Read the model definition and answer for the solid it produces. Units are mm, in the model's axes. Face numbers are marked on the shaded views. A direction names the side the tool comes from. Coordinates: 2 decimals unless noted, no trailing zeros. Write each loop counter-clockwise with the first axis right and the second up, starting at its lowest first coordinate (ties: lowest second). Pieces come first, ordered by that corner, then holes. Notation, with made-up numbers: (39.5, -1) -> (58.5, -1) arc R19 cw to (58.5, 36) -> close; hole circle Ø7 at (73.25, 55). An arc over 180 degrees is marked (long way). Answer as a JSON object with one key per item and string values. Group by question number.
(1) Find section B-B (z = 12.5). Give the vertices of the cut face in (x, y).
(2) Flat-ended cylindrical pins translate along their axes: P1, Ø12, axis at x = 38, z = 14.5, coming from the +Y side; P2, Ø6, axis at x = -20.5, y = 8.5, coming from the +Z side; P3, Ø4.5, axis at x = 6, z = -6, coming from the +Y side. Find the tip coordinate at first contact, or state that the pin passes through.
(3) Which of the six approach directions +Z, -Z, +X, -X, +Y, -Y give full straight-line access (tool end or side, diameter ignored) to the marked faces 5, 6, 7, 8 and 9?
(4) For a pull along X with two mould halves and no side action, classify the marked faces 1, 2, 3 and 4 as +X half, -X half, draft (parallel to the pull), parting line (faces both ways), or undercut.
(5) Straight lines are drawn through the part: L1, parallel to X at y = 15, z = -7; L2, parallel to X at y = 17, z = -8.5; L3, parallel to X at y = 1.5, z = -0.5. For each, find the intervals that lie inside material, in ascending order.
(6) Find section C-C (y = -24). Give the vertices of the cut face in (x, z), then the cut area to 3 significant figures.
(7) Find section D-D (y = 15). Give the vertices of the cut face in (x, z).
(8) Find section A-A (x = -37.5). Give the vertices of the cut face in (y, z), then the cut area to 3 significant figures.
from build123d import *

# Parameters (mm, degrees)
BOSS_EXTRUDE1_DEPTH = 15
SKETCH2_W           = 25
SKETCH2_H           = 10
BOSS_EXTRUDE2_DEPTH = 25
SKETCH3_R           = 2
CUT_EXTRUDE1_DEPTH  = 10


with BuildPart() as part:
    # Sketch1 → Boss-Extrude1 (new body)
    with BuildSketch(Plane.XY):
        with BuildLine():
            Line((-15, 0), (0, 0))
            Line((0, 0), (15, 0))
            Line((15, 0), (15, 30))
            Line((15, 30), (26.540029545, 30))
            Line((26.540029545, 30), (26.540029545, 18.872983346))
            ThreePointArc((26.540029545, 18.872983346), (27.540029545, 11), (28.540029545, 18.872983346))
            Line((28.540029545, 18.872983346), (28.540029545, 30))
            Line((28.540029545, 30), (40, 30))
            Line((40, 30), (40, 0))
            Line((40, 0), (50, -20))
            Line((50, -20), (50, -30))
            Line((50, -30), (0, -30))
            Line((0, -30), (-50, -30))
            Line((-50, -30), (-50, -20))
            Line((-50, -20), (-40, 0))
            Line((-40, 0), (-40, 30))
            Line((-40, 30), (-28.459970455, 30))
            Line((-28.459970455, 30), (-28.459970455, 18.872983346))
            ThreePointArc((-28.459970455, 18.872983346), (-27.459970455, 11), (-26.459970455, 18.872983346))
            Line((-26.459970455, 18.872983346), (-26.459970455, 30))
            Line((-26.459970455, 30), (-15, 30))
            Line((-15, 30), (-15, 0))
        make_face()
    extrude(amount=-BOSS_EXTRUDE1_DEPTH)

    # Sketch2 → Boss-Extrude2 (add)
    with BuildSketch(Plane.XY):
        with Locations((-37.5, -25)):
            Rectangle(SKETCH2_W, SKETCH2_H)
        with Locations((37.5, -25)):
            Rectangle(SKETCH2_W, SKETCH2_H)
    extrude(amount=BOSS_EXTRUDE2_DEPTH)

    # Sketch3 → Cut-Extrude1 (cut)
    with BuildSketch(Plane(origin=(0, -20, 0), x_dir=(1, 0, 0), z_dir=(0, 1, 0))):
        with Locations(Location((-37.5, -12.5, 0), (0, 0, 270))):
            Circle(SKETCH3_R)
        with Locations(Location((37.5, -12.5, 0), (0, 0, 270))):
            Circle(SKETCH3_R)
    extrude(amount=-CUT_EXTRUDE1_DEPTH, mode=Mode.SUBTRACT)


solid = part.part
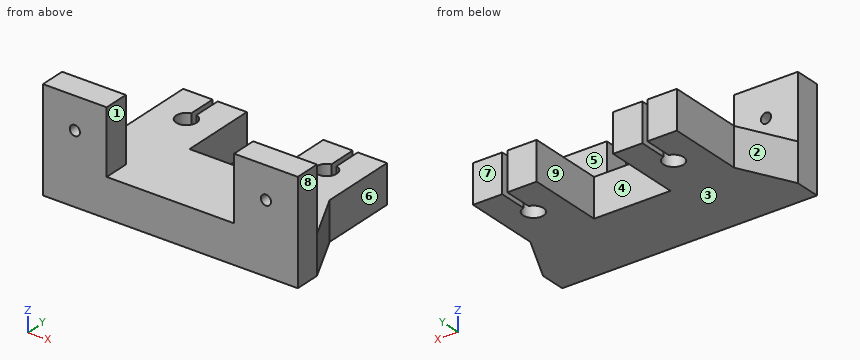
Results below:
{
 "1": {"outline": "(-50, -30) -> (-39.5, -30) -> (-39.5, -20) -> (-50, -20) -> close; (-35.5, -30) -> (-25, -30) -> (-25, -20) -> (-35.5, -20) -> close; (25, -30) -> (35.5, -30) -> (35.5, -20) -> (25, -20) -> close; (39.5, -30) -> (50, -30) -> (50, -20) -> (39.5, -20) -> close"},
 "2": {"P1": "stops at y = -20", "P2": "stops at z = 0", "P3": "stops at y = 0"},
 "3": {"face 5": "+Z, +X, -X, +Y", "face 6": "+Z, -Z, +X, +Y", "face 7": "+Z, -Z, +X, -X, +Y", "face 8": "+Z, -Z, +X, +Y, -Y", "face 9": "+Z, -Z, +Y"},
 "4": {"face 1": "undercut", "face 2": "-X half", "face 3": "draft", "face 4": "undercut"},
 "5": {"L1": "x = -40 to -31.46, -23.46 to -15, 15 to 23.54, 31.54 to 40", "L2": "x = -40 to -30.92, -24 to -15, 15 to 24.08, 31 to 40", "L3": "x = -40 to -15, 15 to 40"},
 "6": {"outline": "(-50, -15) -> (50, -15) -> (50, 25) -> (25, 25) -> (25, 0) -> (-25, 0) -> (-25, 25) -> (-50, 25) -> close; hole circle Ø4 at (-37.5, 12.5); hole circle Ø4 at (37.5, 12.5)", "area": "2,720 mm2"},
 "7": {"outline": "(-40, -15) -> (-31.46, -15) -> (-31.46, 0) -> (-40, 0) -> close; (-23.46, -15) -> (-15, -15) -> (-15, 0) -> (-23.46, 0) -> close; (15, -15) -> (23.54, -15) -> (23.54, 0) -> (15, 0) -> close; (31.54, -15) -> (40, -15) -> (40, 0) -> (31.54, 0) -> close"},
 "8": {"outline": "(-30, -15) -> (30, -15) -> (30, 0) -> (-20, 0) -> (-20, 10.5) -> (-30, 10.5) -> close; (-30, 14.5) -> (-20, 14.5) -> (-20, 25) -> (-30, 25) -> close", "area": "1,110 mm2"}
}
